```python
from build123d import *

# Parameters (mm, degrees)
SM_BASE_FLANGE_1_DEPTH = 6


# Sheet-metal steps are written as plain solids
with BuildPart() as part:
    # Sketch 1 → Базовая кромка1 (new body)
    with BuildSketch(Plane(origin=(0, 0, 0), x_dir=(0, 0, -1), z_dir=(1, 0, 0))):
        with BuildLine():
            Line((250, -150), (-250, -150))
            Line((-250, -150), (-143.570968245, -45.596595724))
            Line((-143.570968245, -45.596595724), (-104.305880907, -37.964235909))
            ThreePointArc((-104.305880907, -37.964235909), (0, -111), (104.305880907, -37.964235909))
            Line((104.305880907, -37.964235909), (143.570968245, -45.596595724))
            Line((143.570968245, -45.596595724), (250, -150))
        make_face()
    extrude(amount=-SM_BASE_FLANGE_1_DEPTH)


solid = part.part
```
Could you check a few things on this model? Use its own coordinates, in mm. Coordinates: 2 decimals unless noted, no trailing zeros. Loops run counter-clockwise (first coordinate to the right, second up) from the corner with the lowest first, then second, coordinate; pieces in that order, holes last.
1) Will these pins go through, and if not, where does the flat tip stop? pin 1 Ø2 at (x, z) = (-4, -118) entering from +Y; pin 2 Ø3 at (x, y) = (-3.5, -128) entering from +Z; pin 3 Ø1 at (x, y) = (-4.5, -110) entering from -Z.
Reported:
pin 1: stops at y = -40.43
pin 2: stops at z = 229.1
pin 3: stops at z = -209.73
2) Please list where these lines run through material, in increasing order: line 1 along Z through (x, y) = (-3.25, -90.5); line 2 along Z through (x, y) = (-3, -53.5); line 3 along Y through (x, z) = (-3.6, 36).
Reported:
line 1: z = -189.35 to -64.27, 64.27 to 189.35
line 2: z = -151.63 to -97.26, 97.26 to 151.63
line 3: y = -150 to -105
3) Imagine slicing it at C-C (y = -58). List the corners of the cut face in (x, z) for me.
Reported:
outline: (-6, -156.22) - (0, -156.22) - (0, -94.64) - (-6, -94.64) - close; (-6, 94.64) - (0, 94.64) - (0, 156.22) - (-6, 156.22) - close
4) Imagine slicing it at A-A (y = -92). List the corners of the cut face in (x, z) for me.
Reported:
outline: (-6, -190.87) - (0, -190.87) - (0, -62.1) - (-6, -62.1) - close; (-6, 62.1) - (0, 62.1) - (0, 190.87) - (-6, 190.87) - close
5) Imagine slicing it at D-D (z = 214). List the corners of the cut face in (x, y) for me.
Reported:
outline: (-6, -150) - (0, -150) - (0, -114.69) - (-6, -114.69) - close
6) Imagine slicing it at B-B (x = -2.5). List the corners of the cut face in (y, z) for me.
Reported:
outline: (-150, -250) - (-45.6, -143.57) - (-37.96, -104.31) arc R111 cw to (-37.96, 104.31) - (-45.6, 143.57) - (-150, 250) - close
7) Thinking about a two-plate mould opening in Z: for faces 1 (the face through (-2.958, -97.067, -196.04)), 2 (the face through (-2.958, -110.984, 1.898)), 3 (the face through (0, -118, -3)), which applies, released by +Z, released by -Z, zero draft, split by the parting line, or undercut?
Reported:
face 1: released by -Z
face 2: undercut
face 3: zero draft
